Read the model definition and answer for the solid it produces. Units are mm, in the model's axes. A direction names the side the tool comes from. Coordinates: 2 decimals unless noted, no trailing zeros. Order: outer loops, then holes, each group sorted by start corner. A loop starts at its lowest first (then second) coordinate and runs counter-clockwise, first axis right, second up. Notation, with made-up numbers: M 61.5,-21 L 86.5,-21 A27 cw 86.5,-1 Z; hole C 76.5,53.5 d7. An arc over 180 degrees is marked long. Use a Markdown table: item, result. Add a question column.
1) Find section A-A on z = 8.5. Write down the section's boundary in (x, y).
2) Find section D-D on y = -6. Write down the section's boundary in (x, z), plus the area to 3 significant figures.
3) The mould has two halves that part along Y. Classify faces 1 (the face through (8.91, 33.46, 5.44)), 2 (the face through (10.11, 14.42, 5.44)), 3 (the face through (10.09, 4.54, 5.44)): released by +Y, released by -Y, zero draft, split by the parting line, or undercut.
4) For faces 4 (the face through (8.89, 23.58, 5.44)), 5 (the face through (8.088, 10, 5)), 6 (the face through (10.912, 9, 5)), 7 (the face through (10.11, 33.42, 5.44)), determine the directions among +Z, -Z, +X, -X, +Y, -Y from which every point of the face is accessible in a straight line to the end or side of a thin tool.
5) Each of these flat-tipped pins is pushed along its axis until it touches: pin 1 Ø5 at (y, z) = (27, 6) entering from +X; pin 2 Ø5 at (y, z) = (4.5, 8) entering from -X. Where does it stop, or does it pass through?
6) Find section C-C on x = -58. Write down the section's boundary in (y, z), plus the area to 3 significant figures.
7) Find the intervals of material crossed by probe 1 along X at (y, z) = (30, 3.75); probe 2 along Z at (x, y) = (-21, 13); probe 3 along X at (y, z) = (23, 6), in increasing order. Write a range as [from, to].
8) Find section B-B on y = 8. Write down the section's boundary in (x, z).
from build123d import *

# Parameters (mm, degrees)
F0_W     = 59
F0_H     = 62
F0_W_2   = 38
F1_DEPTH = 1
F2_DEPTH = 10
F3_R     = 5


# Not quite as in the source:
# - a feature names something its author has since deleted; it is built from what else it names


with BuildPart() as f1:
    # F0 (on Top) → F1 (new body)
    with BuildSketch(Plane.XY):
        with Locations((-39, 19)):
            Rectangle(F0_W, F0_H)
        with Locations((9.5, 19)):
            Rectangle(F0_W_2, F0_H)
        with BuildLine():
            ThreePointArc((9.5, 15.8775010008), (10.0985618966, 14.4432029131), (10.9121369044, 13.1189736826))
            Line((10.9121369044, 13.1189736826), (10.9121369044, 5.8810263174))
            ThreePointArc((10.9121369044, 5.8810263174), (10.0985618966, 4.5567970869), (9.5, 3.1224989992))
            ThreePointArc((9.5, 3.1224989992), (8.9014381034, 4.5567970869), (8.0878630956, 5.8810263174))
            Line((8.0878630956, 5.8810263174), (8.0878630956, 13.1189736826))
            ThreePointArc((8.0878630956, 13.1189736826), (8.9014381034, 14.4432029131), (9.5, 15.8775010008))
        make_face(mode=Mode.SUBTRACT)
        with BuildLine():
            Line((8.0878630956, 24.8810263174), (8.0878630956, 32.1189736826))
            ThreePointArc((8.0878630956, 32.1189736826), (8.9014381034, 33.4432029131), (9.5, 34.8775010008))
            ThreePointArc((9.5, 34.8775010008), (10.0985618966, 33.4432029131), (10.9121369044, 32.1189736826))
            Line((10.9121369044, 32.1189736826), (10.9121369044, 24.8810263174))
            ThreePointArc((10.9121369044, 24.8810263174), (10.0985618966, 23.5567970869), (9.5, 22.1224989992))
            ThreePointArc((9.5, 22.1224989992), (8.9014381034, 23.5567970869), (8.0878630956, 24.8810263174))
        make_face(mode=Mode.SUBTRACT)
    extrude(amount=F1_DEPTH)

    # F0 (on Top) → F2 (join)
    with BuildSketch(Plane.XY):
        with BuildLine():
            ThreePointArc((9.5, 34.8775010008), (8.9014381034, 33.4432029131), (8.0878630956, 32.1189736826))
            Line((8.0878630956, 32.1189736826), (8.0878630956, 24.8810263174))
            ThreePointArc((8.0878630956, 24.8810263174), (8.9014381034, 23.5567970869), (9.5, 22.1224989992))
            ThreePointArc((9.5, 22.1224989992), (10.0985618966, 23.5567970869), (10.9121369044, 24.8810263174))
            Line((10.9121369044, 24.8810263174), (10.9121369044, 32.1189736826))
            ThreePointArc((10.9121369044, 32.1189736826), (10.0985618966, 33.4432029131), (9.5, 34.8775010008))
        make_face()
        with BuildLine():
            Line((10.9121369044, 5.8810263174), (10.9121369044, 13.1189736826))
            ThreePointArc((10.9121369044, 13.1189736826), (10.0985618966, 14.4432029131), (9.5, 15.8775010008))
            ThreePointArc((9.5, 15.8775010008), (8.9014381034, 14.4432029131), (8.0878630956, 13.1189736826))
            Line((8.0878630956, 13.1189736826), (8.0878630956, 5.8810263174))
            ThreePointArc((8.0878630956, 5.8810263174), (8.9014381034, 4.5567970869), (9.5, 3.1224989992))
            ThreePointArc((9.5, 3.1224989992), (10.0985618966, 4.5567970869), (10.9121369044, 5.8810263174))
        make_face()
    extrude(amount=F2_DEPTH)

    # F3
    f3_edges = [f1.edges().sort_by_distance(p)[0] for p in [
        (-68.5, 50, 0.5),
        (28.5, 50, 0.5),
        (28.5, -12, 0.5),
        (-68.5, -12, 0.5),
    ]]
    fillet(f3_edges, radius=F3_R)


solid = f1.part
Check result:
| question | item | result |
|---|---|---|
| 1 | outline | M 8.09,5.88 A10 cw 9.5,3.12 A10 cw 10.91,5.88 L 10.91,13.12 A10 cw 9.5,15.88 A10 cw 8.09,13.12 Z; M 8.09,24.88 A10 cw 9.5,22.12 A10 cw 10.91,24.88 L 10.91,32.12 A10 cw 9.5,34.88 A10 cw 8.09,32.12 Z |
| 2 | outline | M -68.5,0 L 28.5,0 L 28.5,1 L -68.5,1 Z |
| 2 | area | 97.0 mm2 |
| 3 | face 1 | released by +Y |
| 3 | face 2 | undercut |
| 3 | face 3 | released by -Y |
| 4 | face 4 | +Z, -X |
| 4 | face 5 | +Z, -X, +Y, -Y |
| 4 | face 6 | +Z, +X, +Y, -Y |
| 4 | face 7 | +Z, +X, +Y |
| 5 | pin 1 | stops at x = 10.91 |
| 5 | pin 2 | stops at x = 8.09 |
| 6 | outline | M -12,0 L 50,0 L 50,1 L -12,1 Z |
| 6 | area | 62.0 mm2 |
| 7 | probe 1 | x = [8.09, 10.91] |
| 7 | probe 2 | z = [0, 1] |
| 7 | probe 3 | x = [9.17, 9.83] |
| 8 | outline | M -68.5,0 L 28.5,0 L 28.5,1 L 10.91,1 L 10.91,10 L 8.09,10 L 8.09,1 L -68.5,1 Z |
